Part print with two shaded views. Sizes in mm from the minimum x, y, z corner. Give positions to 0.01 mm unless a question says otherwise; leave off trailing zeros. Write each loop counter-clockwise with the first axis right and the second up, starting at its lowest first coordinate (ties: lowest second). Pieces come first, ordered by that corner, then holes.
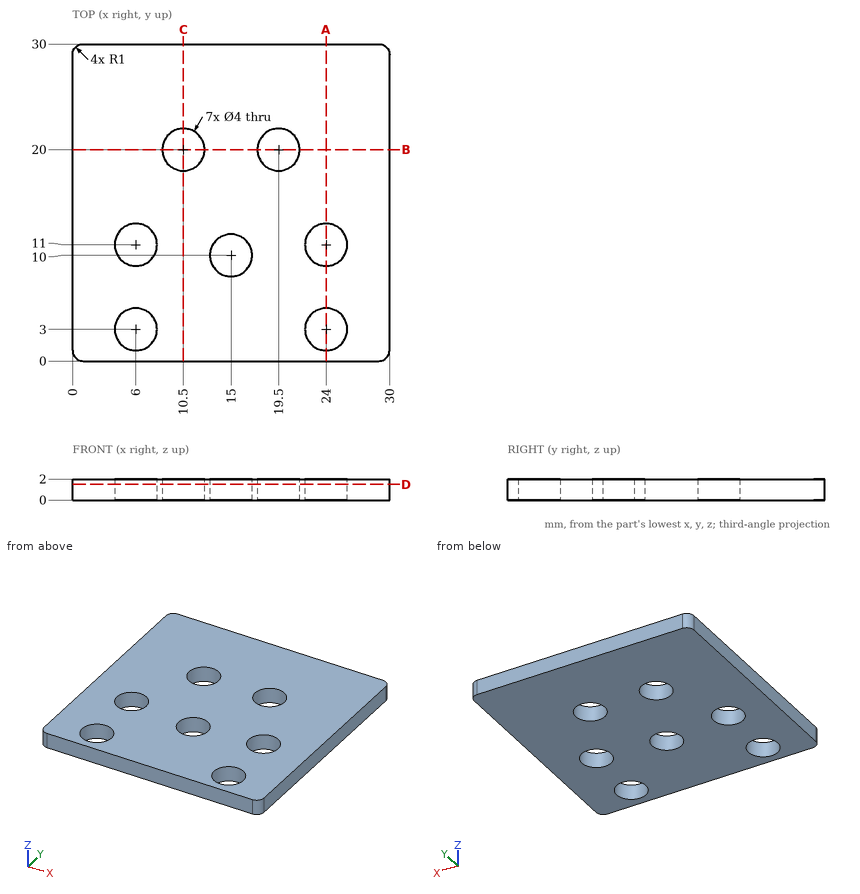
1) Pin check, flat tip, straight feed: pin 1 Ø3 at (x, y) = (6, 11) entering from -Z. Stop position of the tip, or through.
Answers follow:
pin 1: passes through
2) Saw through at B-B, the plane y = 20. Write the cut outline in (x, z), then the cut area to 3 significant figures.
Answers follow:
outline: (0, 0) - (8.5, 0) - (8.5, 2) - (0, 2) - close; (12.5, 0) - (17.5, 0) - (17.5, 2) - (12.5, 2) - close; (21.5, 0) - (30, 0) - (30, 2) - (21.5, 2) - close
area: 44.0 mm2
3) Saw through at A-A, the plane x = 24. Write the cut outline in (y, z).
Answers follow:
outline: (0, 0) - (1, 0) - (1, 2) - (0, 2) - close; (5, 0) - (9, 0) - (9, 2) - (5, 2) - close; (13, 0) - (30, 0) - (30, 2) - (13, 2) - close
4) Saw through at D-D, the plane z = 1.5. Write the cut outline in (x, y).
Answers follow:
outline: (0, 1) arc R1 ccw to (1, 0) - (29, 0) arc R1 ccw to (30, 1) - (30, 29) arc R1 ccw to (29, 30) - (1, 30) arc R1 ccw to (0, 29) - close; hole circle Ø4 at (6, 3); hole circle Ø4 at (6, 11); hole circle Ø4 at (10.5, 20); hole circle Ø4 at (15, 10); hole circle Ø4 at (19.5, 20); hole circle Ø4 at (24, 3); hole circle Ø4 at (24, 11)
5) Saw through at C-C, the plane x = 10.5. Write the cut outline in (y, z).
Answers follow:
outline: (0, 0) - (18, 0) - (18, 2) - (0, 2) - close; (22, 0) - (30, 0) - (30, 2) - (22, 2) - close
6) Wall check: L1, parallel to Y at x = 24, z = 0.8; L2, parallel to Y at x = 10.5, z = 1.75; L3, parallel to Y at x = 7.75, z = 1.9. Give the ranges that are in metal, low to high.
Answers follow:
L1: y = 0 to 1, 5 to 9, 13 to 30
L2: y = 0 to 18, 22 to 30
L3: y = 0 to 2.03, 3.97 to 10.03, 11.97 to 30
